from build123d import *

# Parameters (mm, degrees)
BASE_FLANGE1_DEPTH = 82.5
SKETCH2_R          = 5
CUT_EXTRUDE1_DEPTH = 134.230513755


# Sheet-metal steps are written as plain solids
with BuildPart() as part:
    # Sketch1 → Base-Flange1 (new, symmetric)
    with BuildSketch(Plane.XY):
        with BuildLine():
            Line((-91.891891892, 135), (-79.604112678, 148.777206997))
            ThreePointArc((-79.604112678, 148.777206997), (-78.370281896, 149.6803294), (-76.875029682, 150))
            Line((-76.875029682, 150), (-1, 150))
            ThreePointArc((-1, 150), (-0.292893219, 150.292893219), (0, 151))
            Line((0, 151), (0, 200))
            Line((0, 200), (2.65684, 200))
            Line((2.65684, 200), (2.65684, 151))
            ThreePointArc((2.65684, 151), (1.585776362, 148.414223638), (-1, 147.34316))
            Line((-1, 147.34316), (-76.875029682, 147.34316))
            ThreePointArc((-76.875029682, 147.34316), (-77.28392157, 147.255742831), (-77.621325116, 147.008774847))
            Line((-77.621325116, 147.008774847), (-89.90910433, 133.23156785))
            Line((-89.90910433, 133.23156785), (-91.891891892, 135))
        make_face()
    extrude(amount=BASE_FLANGE1_DEPTH, both=True)

    # Sketch2 → Cut-Extrude1 (cut, through all)
    with BuildSketch(Plane(origin=(0, 150, 0), x_dir=(1, 0, 0), z_dir=(0, 1, 0))):
        with Locations(Location((-66.875029682, 72.5, 0), (0, 0, 270))):
            Circle(SKETCH2_R)
        with Locations(Location((-49.875029682, 72.5, 0), (0, 0, 270))):
            Circle(SKETCH2_R)
        with Locations(Location((-32.875029682, 72.5, 0), (0, 0, 270))):
            Circle(SKETCH2_R)
        with Locations(Location((-15.875029682, 72.5, 0), (0, 0, 270))):
            Circle(SKETCH2_R)
        with Locations(Location((-66.875029682, 56.5, 0), (0, 0, 270))):
            Circle(SKETCH2_R)
        with Locations(Location((-49.875029682, 56.5, 0), (0, 0, 270))):
            Circle(SKETCH2_R)
        with Locations(Location((-32.875029682, 56.5, 0), (0, 0, 270))):
            Circle(SKETCH2_R)
        with Locations(Location((-15.875029682, 56.5, 0), (0, 0, 270))):
            Circle(SKETCH2_R)
        with Locations(Location((-66.875029682, 40.5, 0), (0, 0, 270))):
            Circle(SKETCH2_R)
        with Locations(Location((-49.875029682, 40.5, 0), (0, 0, 270))):
            Circle(SKETCH2_R)
        with Locations(Location((-32.875029682, 40.5, 0), (0, 0, 270))):
            Circle(SKETCH2_R)
        with Locations(Location((-15.875029682, 40.5, 0), (0, 0, 270))):
            Circle(SKETCH2_R)
        with Locations(Location((-66.875029682, 24.5, 0), (0, 0, 270))):
            Circle(SKETCH2_R)
        with Locations(Location((-49.875029682, 24.5, 0), (0, 0, 270))):
            Circle(SKETCH2_R)
        with Locations(Location((-32.875029682, 24.5, 0), (0, 0, 270))):
            Circle(SKETCH2_R)
        with Locations(Location((-15.875029682, 24.5, 0), (0, 0, 270))):
            Circle(SKETCH2_R)
        with Locations(Location((-66.875029682, 8.5, 0), (0, 0, 270))):
            Circle(SKETCH2_R)
        with Locations(Location((-49.875029682, 8.5, 0), (0, 0, 270))):
            Circle(SKETCH2_R)
        with Locations(Location((-32.875029682, 8.5, 0), (0, 0, 270))):
            Circle(SKETCH2_R)
        with Locations(Location((-15.875029682, 8.5, 0), (0, 0, 270))):
            Circle(SKETCH2_R)
        with Locations(Location((-66.875029682, -7.5, 0), (0, 0, 270))):
            Circle(SKETCH2_R)
        with Locations(Location((-49.875029682, -7.5, 0), (0, 0, 270))):
            Circle(SKETCH2_R)
        with Locations(Location((-32.875029682, -7.5, 0), (0, 0, 270))):
            Circle(SKETCH2_R)
        with Locations(Location((-15.875029682, -7.5, 0), (0, 0, 270))):
            Circle(SKETCH2_R)
        with Locations(Location((-66.875029682, -23.5, 0), (0, 0, 270))):
            Circle(SKETCH2_R)
        with Locations(Location((-49.875029682, -23.5, 0), (0, 0, 270))):
            Circle(SKETCH2_R)
        with Locations(Location((-32.875029682, -23.5, 0), (0, 0, 270))):
            Circle(SKETCH2_R)
        with Locations(Location((-15.875029682, -23.5, 0), (0, 0, 270))):
            Circle(SKETCH2_R)
        with Locations(Location((-66.875029682, -39.5, 0), (0, 0, 270))):
            Circle(SKETCH2_R)
        with Locations(Location((-49.875029682, -39.5, 0), (0, 0, 270))):
            Circle(SKETCH2_R)
        with Locations(Location((-32.875029682, -39.5, 0), (0, 0, 270))):
            Circle(SKETCH2_R)
        with Locations(Location((-15.875029682, -39.5, 0), (0, 0, 270))):
            Circle(SKETCH2_R)
        with Locations(Location((-66.875029682, -55.5, 0), (0, 0, 270))):
            Circle(SKETCH2_R)
        with Locations(Location((-49.875029682, -55.5, 0), (0, 0, 270))):
            Circle(SKETCH2_R)
        with Locations(Location((-32.875029682, -55.5, 0), (0, 0, 270))):
            Circle(SKETCH2_R)
        with Locations(Location((-15.875029682, -55.5, 0), (0, 0, 270))):
            Circle(SKETCH2_R)
        with Locations(Location((-66.875029682, -71.5, 0), (0, 0, 270))):
            Circle(SKETCH2_R)
        with Locations(Location((-49.875029682, -71.5, 0), (0, 0, 270))):
            Circle(SKETCH2_R)
        with Locations(Location((-32.875029682, -71.5, 0), (0, 0, 270))):
            Circle(SKETCH2_R)
        with Locations(Location((-15.875029682, -71.5, 0), (0, 0, 270))):
            Circle(SKETCH2_R)
    extrude(amount=-CUT_EXTRUDE1_DEPTH, mode=Mode.SUBTRACT)


solid = part.part
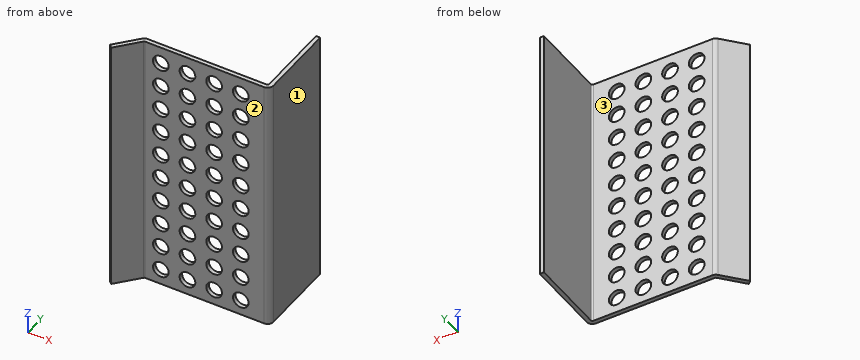
Verification items for the finished model (mm, model axes). Face numbers are marked on the shaded views. A direction names the side the tool comes from. Coordinates: 2 decimals unless noted, no trailing zeros. Order: outer loops, then holes, each group sorted by start corner. A loop starts at its lowest first (then second) coordinate and runs counter-clockwise, first axis right, second up.
Item 1: Section check B-B, the plane x = -12.5. Give the number of separate pieces and of enclosed holes in the cut face, then the cut area to 3 significant figures.
Filled in:
separate pieces: 11
enclosed holes: 0
area: 242 mm2
Item 2: Section check D-D, the plane y = 187. Enter the section's corners in (x, z).
Filled in:
outline: (0, -82.5) - (2.66, -82.5) - (2.66, 82.5) - (0, 82.5) - close
Item 3: Access from +Z, -Z, +X, -X, +Y, -Y to the whole of each face (thin tool, end or side, straight path). Record for the marked faces 1, 2 and 3.
Filled in:
face 1: +Z, -Z, +X, +Y, -Y
face 2: +Z, -Z, +X, -Y
face 3: +Z, -Z, -X, +Y
Item 4: Depth check by flat-ended pin: pin 1 (5 mm diameter, centred on x = -36, z = -31.5, fed in from +Y); pin 2 (5 mm diameter, centred on y = 142.5, z = 8.5, fed in from -X); pin 3 (6 mm diameter, centred on y = 144.5, z = 64.5, fed in from -X); pin 4 (8 mm diameter, centred on x = -15.88, z = -24.5, fed in from +Y). Enter the tip coordinate at first touch or a pass-through.
Filled in:
pin 1: stops at y = 150
pin 2: stops at x = -87.43
pin 3: stops at x = -86.09
pin 4: passes through
Item 5: Material ranges on L1, parallel to X at y = 149.45, z = -40.5; L2, parallel to X at y = 149, z = 55; L3, parallel to X at y = 189, z = -15.5, recorded low to high.
Filled in:
L1: x = -78.8 to -71.88, -61.88 to -54.88, -44.88 to -37.88, -27.88 to -20.88, -10.88 to 2.31
L2: x = -79.39 to -71.85, -61.9 to -54.85, -44.9 to -37.85, -27.9 to -20.85, -10.9 to 2.06
L3: x = 0 to 2.66
Item 6: Section check C-C, the plane z = -11.5. Enter the section's corners in (x, y), then the cut area to 3 significant figures.
Filled in:
outline: (-91.89, 135) - (-89.91, 133.23) - (-77.62, 147.01) arc R1 cw to (-76.88, 147.34) - (-70.88, 147.34) - (-70.88, 150) - (-76.88, 150) arc R3.66 ccw to (-79.6, 148.78) - close; (-62.88, 147.34) - (-53.88, 147.34) - (-53.88, 150) - (-62.88, 150) - close; (-45.88, 147.34) - (-36.88, 147.34) - (-36.88, 150) - (-45.88, 150) - close; (-28.88, 147.34) - (-19.88, 147.34) - (-19.88, 150) - (-28.88, 150) - close; (-11.88, 147.34) - (-1, 147.34) arc R3.66 ccw to (2.66, 151) - (2.66, 200) - (0, 200) - (0, 151) arc R1 cw to (-1, 150) - (-11.88, 150) - close
area: 311 mm2
Item 7: Section check A-A, the plane z = 39.5. Enter the section's corners in (x, y).
Filled in:
outline: (-91.89, 135) - (-89.91, 133.23) - (-77.62, 147.01) arc R1 cw to (-76.88, 147.34) - (-71.88, 147.34) - (-71.88, 150) - (-76.88, 150) arc R3.66 ccw to (-79.6, 148.78) - close; (-61.88, 147.34) - (-54.88, 147.34) - (-54.88, 150) - (-61.88, 150) - close; (-44.88, 147.34) - (-37.88, 147.34) - (-37.88, 150) - (-44.88, 150) - close; (-27.88, 147.34) - (-20.88, 147.34) - (-20.88, 150) - (-27.88, 150) - close; (-10.88, 147.34) - (-1, 147.34) arc R3.66 ccw to (2.66, 151) - (2.66, 200) - (0, 200) - (0, 151) arc R1 cw to (-1, 150) - (-10.88, 150) - close
